```python
from build123d import *

# Parameters (mm, degrees)
BOSS_EXTRUDE1_DEPTH = 25
SKETCH3_W           = 36
SKETCH3_H           = 10
CUT_EXTRUDE1_DEPTH  = 134.88427839
CUT_EXTRUDE2_DEPTH  = 134.88427839
CUT_EXTRUDE3_DEPTH  = 134.88427839
CUT_EXTRUDE4_DEPTH  = 134.88427839
CUT_EXTRUDE5_DEPTH  = 134.88427839
CUT_EXTRUDE6_DEPTH  = 134.88427839
CUT_EXTRUDE7_DEPTH  = 134.88427839
CUT_EXTRUDE8_DEPTH  = 134.88427839
CUT_EXTRUDE9_DEPTH  = 134.88427839
FILLET1_R           = 1
BOSS_EXTRUDE2_DEPTH = 25
BOSS_EXTRUDE3_DEPTH = 25
LPATTERN1_COUNT     = 30
LPATTERN1_PITCH     = 3


with BuildPart() as part:
    # Sketch2 → Boss-Extrude1 (new body)
    with BuildSketch(Plane.XY):
        with BuildLine():
            Line((-15, 0), (15, 0))
            Line((15, 0), (15, 5))
            Line((15, 5), (8, 5))
            Line((8, 5), (8, 10))
            Line((8, 10), (20, 10))
            Line((20, 10), (20, 130))
            ThreePointArc((20, 130), (-9.083269132, 106.055512755), (-20, 70))
            Line((-20, 70), (-20, 10))
            Line((-20, 10), (-8, 10))
            Line((-8, 10), (-8, 5))
            Line((-8, 5), (-15, 5))
            Line((-15, 5), (-15, 0))
        make_face()
    extrude(amount=BOSS_EXTRUDE1_DEPTH)

    # Sketch3 → Cut-Extrude1 (cut, through all)
    with BuildSketch(Plane.XY.offset(25)):
        with Locations((0, 17)):
            Rectangle(SKETCH3_W, SKETCH3_H)
    extrude(amount=-CUT_EXTRUDE1_DEPTH, mode=Mode.SUBTRACT)

    # Sketch4 → Cut-Extrude2 (cut, through all)
    with BuildSketch(Plane.XY.offset(25)):
        Polygon((-18, 23), (18, 23), (18, 33), (-18, 39.347771306), align=None)
    extrude(amount=-CUT_EXTRUDE2_DEPTH, mode=Mode.SUBTRACT)

    # Sketch5 → Cut-Extrude3 (cut, through all)
    with BuildSketch(Plane.XY.offset(25)):
        Polygon((-18, 40.363197917), (18, 34.015426612), (18, 44.015426612), (-18, 57.118355045), align=None)
    extrude(amount=-CUT_EXTRUDE3_DEPTH, mode=Mode.SUBTRACT)

    # Sketch6 → Cut-Extrude4 (cut, through all)
    with BuildSketch(Plane.XY.offset(25)):
        with BuildLine():
            Line((-18, 58.182532818), (18, 45.079604384))
            Line((18, 45.079604384), (18, 55.079604384))
            Line((18, 55.079604384), (-17.740313653, 75.714284093))
            ThreePointArc((-17.740313653, 75.714284093), (-17.935044928, 72.860090894), (-18, 70))
            Line((-18, 70), (-18, 58.182532818))
        make_face()
    extrude(amount=-CUT_EXTRUDE4_DEPTH, mode=Mode.SUBTRACT)

    # Sketch12 → Cut-Extrude5 (cut, through all)
    with BuildSketch(Plane.XY.offset(25)):
        with BuildLine():
            Line((-17.631285006, 76.806036913), (18, 56.234304923))
            Line((18, 56.234304923), (18, 66.234304923))
            Line((18, 66.234304923), (-13.712387619, 92.844157678))
            ThreePointArc((-13.712387619, 92.844157678), (-16.199485709, 84.954027852), (-17.631285006, 76.806036913))
        make_face()
    extrude(amount=-CUT_EXTRUDE5_DEPTH, mode=Mode.SUBTRACT)

    # Sketch7 → Cut-Extrude6 (cut, through all)
    with BuildSketch(Plane.XY.offset(25)):
        with BuildLine():
            Line((-13.322364363, 93.822296597), (18, 67.539712212))
            Line((18, 67.539712212), (18, 77.539712212))
            Line((18, 77.539712212), (-6.326939086, 106.531429264))
            ThreePointArc((-6.326939086, 106.531429264), (-10.191692762, 100.378891521), (-13.322364363, 93.822296597))
        make_face()
    extrude(amount=-CUT_EXTRUDE6_DEPTH, mode=Mode.SUBTRACT)

    # Sketch8 → Cut-Extrude7 (cut, through all)
    with BuildSketch(Plane.XY.offset(25)):
        with BuildLine():
            Line((-5.722234691, 107.366494456), (18, 79.095436039))
            Line((18, 79.095436039), (18, 89.095436039))
            Line((18, 89.095436039), (2.287500379, 116.310283697))
            ThreePointArc((2.287500379, 116.310283697), (-1.93090917, 112.029629602), (-5.722234691, 107.366494456))
        make_face()
    extrude(amount=-CUT_EXTRUDE7_DEPTH, mode=Mode.SUBTRACT)

    # Sketch9 → Cut-Extrude8 (cut, through all)
    with BuildSketch(Plane.XY.offset(25)):
        with BuildLine():
            Line((3.04523541, 116.997848123), (18, 91.095436039))
            Line((18, 91.095436039), (18, 101.095436039))
            Line((18, 101.095436039), (10.202779023, 122.518124607))
            ThreePointArc((10.202779023, 122.518124607), (6.524875761, 119.886519369), (3.04523541, 116.997848123))
        make_face()
    extrude(amount=-CUT_EXTRUDE8_DEPTH, mode=Mode.SUBTRACT)

    # Sketch10 → Cut-Extrude9 (cut, through all)
    with BuildSketch(Plane.XY.offset(25)):
        with BuildLine():
            Line((11.063128519, 123.078138194), (18, 104.019240439))
            Line((18, 104.019240439), (18, 126.920997883))
            ThreePointArc((18, 126.920997883), (14.471038847, 125.108824438), (11.063128519, 123.078138194))
        make_face()
    extrude(amount=-CUT_EXTRUDE9_DEPTH, mode=Mode.SUBTRACT)

    # Fillet1
    fillet1_edges = [part.edges().sort_by_distance(p)[0] for p in [
        (-17.631285006, 76.806036913, 12.5),
        (-13.712387619, 92.844157678, 12.5),
        (18, 66.234304923, 12.5),
        (18, 56.234304923, 12.5),
        (-13.322364363, 93.822296597, 12.5),
        (-6.326939086, 106.531429264, 12.5),
        (18, 77.539712212, 12.5),
        (18, 67.539712212, 12.5),
        (-5.722234691, 107.366494456, 12.5),
        (2.287500379, 116.310283697, 12.5),
        (18, 89.095436039, 12.5),
        (18, 79.095436039, 12.5),
        (3.04523541, 116.997848123, 12.5),
        (10.202779023, 122.518124607, 12.5),
        (18, 101.095436039, 12.5),
        (18, 91.095436039, 12.5),
        (11.063128519, 123.078138194, 12.5),
        (18, 126.920997883, 12.5),
        (18, 104.019240439, 12.5),
        (-18, 12, 12.5),
        (-18, 22, 12.5),
        (18, 22, 12.5),
        (18, 12, 12.5),
        (-18, 23, 12.5),
        (-18, 39.347771306, 12.5),
        (18, 33, 12.5),
        (18, 23, 12.5),
        (-18, 40.363197917, 12.5),
        (-18, 57.118355045, 12.5),
        (18, 44.015426612, 12.5),
        (18, 34.015426612, 12.5),
        (-18, 58.182532818, 12.5),
        (-17.740313653, 75.714284093, 12.5),
        (18, 55.079604384, 12.5),
        (18, 45.079604384, 12.5),
    ]]
    fillet(fillet1_edges, radius=FILLET1_R)

    # Sketch13 → Boss-Extrude2 (add)
    with BuildSketch(Plane.XY.offset(25)):
        with BuildLine():
            Line((28.543587015, 132.015112463), (28.543587015, 130.015112463))
            ThreePointArc((28.543587015, 130.015112463), (22.183163486, 116.610368534), (20, 101.934676234))
            Line((20, 101.934676234), (20, 130))
            ThreePointArc((20, 130), (24.189413282, 131.356828362), (28.543587015, 132.015112463))
        make_face()
    extrude(amount=-BOSS_EXTRUDE2_DEPTH)

    # Sketch15 → Boss-Extrude3 (add)
    with BuildSketch(Plane.XY.offset(25)):
        Polygon((20, 101.934676234), (22.598076211, 100.434676234), (20, 98.934676234), align=None)
    boss_extrude3 = extrude(amount=-BOSS_EXTRUDE3_DEPTH)

    # LPattern1: Boss-Extrude3 ×30
    with Locations(*[(0, -i * LPATTERN1_PITCH, 0) for i in range(1, LPATTERN1_COUNT)]):
        add(boss_extrude3)


solid = part.part
```
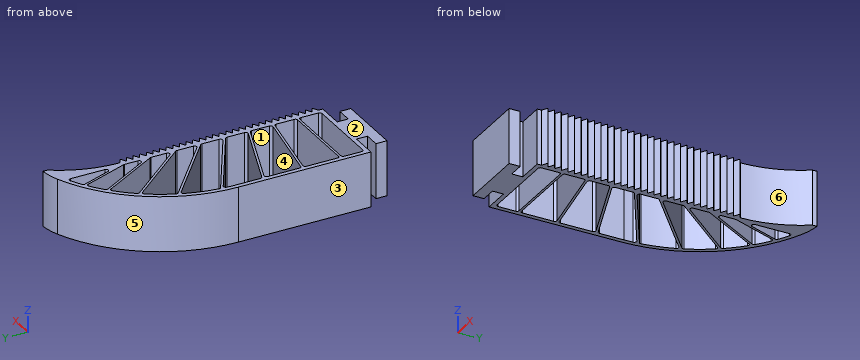
Build history of the part. All positions in model axes, mm. Face numbers are marked on the shaded views. A direction names the side the tool comes from. Round coordinates to 2 decimals unless told otherwise and drop trailing zeros. Order: outer loops, then holes, each group sorted by start corner. A loop starts at its lowest first (then second) coordinate and runs counter-clockwise, first axis right, second up. Notation, with made-up numbers: (41, -4) -> (65, -4) arc R28 ccw to (65, 14) -> close; hole circle Ø3 at (-3, 11.25). An arc over 180 degrees is marked (long way). Answer in a Markdown table with one row per item.
1) Wall check: L1, parallel to X at y = 76.5, z = 4; L2, parallel to X at y = 88.5, z = 20.5; L3, parallel to X at y = 58, z = 19. Give the ranges that are in metal, low to high.
Values:
| item | result |
|---|---|
| L1 | -19.67 to -17.1, 5.77 to 7.32, 18 to 22.48 |
| L2 | -17.31 to -15.22, -8.54 to -6.98, 8.8 to 10.11, 18 to 22.48 |
| L3 | -20 to -17.47, 12.94 to 14.94, 18 to 21.85 |
2) Band-saw the part on A-A on x = -11. Give the number of separate pieces and of enclosed holes in the cut face, and give its area (3 significant figures).
Values:
| item | result |
|---|---|
| separate pieces | 8 |
| enclosed holes | 0 |
| area | 417 mm2 |
3) Which spindle directions (+Z, -Z, +X, -X, +Y, -Y) get a long thin tool onto all of the face, cutting with end or side? Do the marked faces 4, 5 and 6. Say none if no direction does.
Values:
| item | result |
|---|---|
| face 4 | +Z, -Z |
| face 5 | +Z, -Z, -X, +Y |
| face 6 | +Z, -Z, +X |
4) Mould opens along X. For the marked faces 1, 2 and 3 say: released by +X, released by -X, zero draft, split by the parting line, or undercut.
Values:
| item | result |
|---|---|
| face 1 | undercut |
| face 2 | zero draft |
| face 3 | released by -X |
5) Pin check, flat tips, straight feed: P1, Ø7.5, axis at x = -11.5, z = 17.5, coming from the +Y side; P2, Ø0.6, axis at y = 11, z = 15.5, coming from the +X side; P3, Ø10, axis at y = 82.5, z = 4.5, coming from the -X side. Stop position of each tip, or through.
Values:
| item | result |
|---|---|
| P1 | y = 107.98 |
| P2 | x = 20 |
| P3 | x = -19.57 |
6) Band-saw the part on C-C on x = 25. Give the cut face in (y, z).
Values:
| item | result |
|---|---|
| outline | (123.82, 0) -> (131.53, 0) -> (131.53, 25) -> (123.82, 25) -> close |
